Input: part model. Units: mm. Frame: model coordinates. A direction names the side the tool comes from. Give positions to 0.01 mm unless a question says otherwise; leave off trailing zeros. Loops run counter-clockwise (first coordinate to the right, second up) from the corner with the lowest first, then second, coordinate; pieces in that order, holes last. Notation, with made-up numbers: M -38.75,41.5 L 12.25,41.5 A20 ccw 12.25,51.5 Z; hole C 24.5,-18 d1. An arc over 180 degrees is marked long. Answer as a JSON object with one key per item and string values. Group by question number.
1) First-contact query: P1, Ø1.5, axis at y = 1, z = 6.5, coming from the +X side; P2, Ø1, axis at x = 8.5, y = 1, coming from the -Z side. Flat tips, straight axial feed; report the tip coordinate or a pass-through.
2) Ray query, L1, parallel to Z at x = 8, y = 0.6; L2, parallel to X at y = 2.05, z = -8; L3, parallel to Z at x = -26, y = 2.35. Return the intervals inside material, ascending.
3) Section query C-C on z = -48.5. Return loops of the section in (x, y), plus the area to 3 significant figures.
4) Section query A-A on x = -34. Return loops of the section in (y, z).
5) Draft query along X for faces 1 (the cylindrical face through (-33.04, 1.49, -6.37)), 2 (the flat face through (15, 3.02, 4)), 3 (the cylindrical face through (-17.485, 1.531, 8.813)). Return one class per face: +X half, -X half, draft (parallel to the pull), parting line (faces both ways), or undercut.
6) Section query B-B on z = 37.5. Return loops of the section in (x, y).
7) Section query D-D on y = 2.4. Count the separate pieces of the cut face and the enclosed holes in it, plus the area to 3 significant figures.
8) Access query for faces 4 (the flat face through (-23.245, 1.489, -86.689)), 5 (the cylindrical face through (1.012, 1.489, 71.593)), 6 (the cylindrical face through (36.18, 1.53, 11.6)). Directions: +Z, -Z, +X, -X, +Y, -Y. A direction counts if a zero-diameter tool reaches every point of the face in a straight line with its end or side. Return the directions, or none.
from build123d import *

# Parameters (mm, degrees)
BOSS_EXTRUDE1_DEPTH = 3.02
CUT_EXTRUDE2_DEPTH  = 4.02
FILLET6_R           = 5
SKETCH7_R           = 25
BOSS_EXTRUDE5_DEPTH = 3.02
FILLET7_R           = 5
SKETCH8_R           = 11.6
CUT_EXTRUDE3_DEPTH  = 4.0200001
SKETCH10_R          = 2.5
CUT_EXTRUDE4_DEPTH  = 4.0200001


with BuildPart() as part:
    # Sketch1 → Boss-Extrude1 (new body)
    with BuildSketch(Plane(origin=(0, 0, 0), x_dir=(1, 0, 0), z_dir=(0, 1, 0))):
        with BuildLine():
            Line((-29.785324721, 97.135958487), (-16.519810347, 75.945721858))
            ThreePointArc((-16.519810347, 75.945721858), (-15.347350146, 70.779086196), (-17.648053563, 66.006712491))
            ThreePointArc((-17.648053563, 66.006712491), (-19.388749036, 63.401577615), (-20, 60.328611505))
            Line((-20, 60.328611505), (-20, 39.154861291))
            ThreePointArc((-20, 39.154861291), (-33.397395417, 5.995144025), (-66.069350322, -8.551347504))
            Line((-66.069350322, -8.551347504), (-71.066304458, -8.725844988))
            ThreePointArc((-71.066304458, -8.725844988), (2.498803964, -71.556383215), (71.501874688, -3.747254467))
            Line((71.501874688, -3.747254467), (66.504920553, -3.921751951))
            ThreePointArc((66.504920553, -3.921751951), (33.721031142, 8.662804123), (20, 40.987527801))
            Line((20, 40.987527801), (20, 60.328611505))
            ThreePointArc((20, 60.328611505), (4.388325927, 91.285675923), (-29.785324721, 97.135958487))
        make_face()
    extrude(amount=BOSS_EXTRUDE1_DEPTH)

    # Sketch6 → Cut-Extrude2 (cut, through all)
    with BuildSketch(Plane(origin=(0, 3.02, 0), x_dir=(1, 0, 0), z_dir=(0, 1, 0))):
        with BuildLine():
            ThreePointArc((-45.588380428, -19.541227443), (1.807988114, -49.567037222), (46.890896023, -16.167989057))
            ThreePointArc((46.890896023, -16.167989057), (28.340616971, -6.479645741), (14.25203647, 8.995778278))
            ThreePointArc((14.25203647, 8.995778278), (3.327119381, -16.521950459), (-16.623047064, 2.77828664))
            ThreePointArc((-16.623047064, 2.77828664), (-29.443436546, -10.538704339), (-45.588380428, -19.541227443))
        make_face()
    extrude(amount=-CUT_EXTRUDE2_DEPTH, mode=Mode.SUBTRACT)

    # Fillet6
    fillet6_edges = [part.edges().sort_by_distance(p)[0] for p in [
        (-45.588380428, 1.51, 19.541227443),
        (46.890896023, 1.51, 16.167989057),
    ]]
    fillet(fillet6_edges, radius=FILLET6_R)

    # Sketch7 → Boss-Extrude5 (add)
    with BuildSketch(Plane(origin=(0, 3.02, 0), x_dir=(1, 0, 0), z_dir=(0, 1, 0))):
        Circle(SKETCH7_R)
    extrude(amount=-BOSS_EXTRUDE5_DEPTH)

    # Fillet7
    fillet7_edges = [part.edges().sort_by_distance(p)[0] for p in [
        (24.755757684, 1.51, 3.486038077),
        (-24.252747569, 1.51, 6.066649432),
    ]]
    fillet(fillet7_edges, radius=FILLET7_R)

    # Sketch8 → Cut-Extrude3 (cut, through all)
    with BuildSketch(Plane(origin=(0, 3.02, 0), x_dir=(1, 0, 0), z_dir=(0, 1, 0))):
        with Locations((0.168160547, -0.172559626)):
            Circle(SKETCH8_R)
    extrude(amount=-CUT_EXTRUDE3_DEPTH, mode=Mode.SUBTRACT)

    # Sketch10 → Cut-Extrude4 (cut, through all)
    with BuildSketch(Plane(origin=(0, 3.02, 0), x_dir=(1, 0, 0), z_dir=(0, 1, 0))):
        with Locations((0.168160547, -17.672559626)):
            Circle(SKETCH10_R)
        with Locations((-14.987284019, -8.922559626)):
            Circle(SKETCH10_R)
        with Locations((-14.987284019, 8.577440374)):
            Circle(SKETCH10_R)
        with Locations((0.168160547, 17.327440374)):
            Circle(SKETCH10_R)
        with Locations((15.323605113, 8.577440374)):
            Circle(SKETCH10_R)
        with Locations((15.323605113, -8.922559626)):
            Circle(SKETCH10_R)
    extrude(amount=-CUT_EXTRUDE4_DEPTH, mode=Mode.SUBTRACT)


solid = part.part
Output:
{
 "1": {"P1": "stops at x = 71.37", "P2": "stops at z = -88.26"},
 "2": {"L1": "z = -88.26 to -8.38, 8.73 to 23.69, 48.95 to 71.15", "L2": "x = -31.57 to -17.42, -12.55 to -8.06, 8.4 to 12.89, 17.76 to 34.42", "L3": "z = -98.09 to -91.09, -15.99 to 9.44, 42.24 to 66.71"},
 "3": {"outline": "M -20,0 L 20,0 L 20,3.02 L -20,3.02 Z", "area": "121 mm^2"},
 "4": {"outline": "M 0,-5.38 L 3.02,-5.38 L 3.02,13.74 L 0,13.74 Z; M 0,36.11 L 3.02,36.11 L 3.02,63.01 L 0,63.01 Z"},
 "5": {"face 1": "-X half", "face 2": "draft", "face 3": "undercut"},
 "6": {"outline": "M -60.99,0 L -32.46,0 L -32.46,3.02 L -60.99,3.02 Z; M 32.46,0 L 60.99,0 L 60.99,3.02 L 32.46,3.02 Z"},
 "7": {"separate pieces": "1", "enclosed holes": "8", "area": "9,220 mm^2"},
 "8": {"face 4": "-X, +Y, -Y", "face 5": "+Z, +Y, -Y", "face 6": "+Y, -Y"}
}
